```python
from build123d import *

# Parameters (mm, degrees)
ESBO_O1_R                = 14.5
RESSALTO_EXTRUS_O1_DEPTH = 17
ESBO_O1_4_R              = 14.5
ESBO_O1_4_R_2            = 4
RESSALTO_EXTRUS_O2_DEPTH = 13
RESSALTO_EXTRUS_O3_DEPTH = 5
ESBO_O1_9_R              = 4
RESSALTO_EXTRUS_O4_DEPTH = 2


with BuildPart() as part:
    # Esboço1 → Ressalto-extrusão1 (new, symmetric)
    with BuildSketch(Plane.XY):
        with BuildLine():
            ThreePointArc((-16.377431433, -13), (-16.816771262, -14.060660172), (-17.877431433, -14.5))
            Line((-17.877431433, -14.5), (-93.857447864, -14.5))
            Line((-93.857447864, -14.5), (-94.796189578, -14.5))
            ThreePointArc((-94.796189578, -14.5), (-142.377431433, 0), (-94.796189578, 14.5))
            Line((-94.796189578, 14.5), (-93.857447864, 14.5))
            Line((-93.857447864, 14.5), (-17.877431433, 14.5))
            ThreePointArc((-17.877431433, 14.5), (-16.816771262, 14.060660172), (-16.377431433, 13))
            Line((-16.377431433, 13), (-16.377431433, -13))
        make_face()
        with Locations((-116.377431433, 0)):
            Circle(ESBO_O1_R, mode=Mode.SUBTRACT)
        with BuildLine():
            ThreePointArc((-67.404246513, -2), (-55.027431433, 0), (-67.404246513, 2))
            Line((-67.404246513, 2), (-72.243354514, 2))
            Line((-72.243354514, 2), (-72.243354514, -2))
            Line((-72.243354514, -2), (-67.404246513, -2))
        make_face(mode=Mode.SUBTRACT)
    extrude(amount=RESSALTO_EXTRUS_O1_DEPTH, both=True)

    # Esboço1<4> → Ressalto-extrusão2 (add, symmetric)
    # profile 1 of 3: a face of its own
    with BuildSketch(Plane.XY):
        with BuildLine():
            Line((-17.877431433, 14.5), (-93.857447864, 14.5))
            Line((-93.857447864, 14.5), (-94.796189578, 14.5))
            ThreePointArc((-94.796189578, 14.5), (-142.377431433, 0), (-94.796189578, -14.5))
            Line((-94.796189578, -14.5), (-93.857447864, -14.5))
            Line((-93.857447864, -14.5), (-17.877431433, -14.5))
            ThreePointArc((-17.877431433, -14.5), (-16.816771262, -14.060660172), (-16.377431433, -13))
            Line((-16.377431433, -13), (-16.377431433, 13))
            ThreePointArc((-16.377431433, 13), (-16.816771262, 14.060660172), (-17.877431433, 14.5))
        make_face()
        with Locations((-116.377431433, 0)):
            Circle(ESBO_O1_4_R, mode=Mode.SUBTRACT)
        with BuildLine():
            ThreePointArc((-67.404246513, 2), (-55.027431433, 0), (-67.404246513, -2))
            Line((-67.404246513, -2), (-72.243354514, -2))
            Line((-72.243354514, -2), (-72.243354514, 2))
            Line((-72.243354514, 2), (-67.404246513, 2))
        make_face(mode=Mode.SUBTRACT)
    # profile 2 of 3: a face of its own
    with BuildSketch(Plane.XY):
        Polygon((-1.377431433, 13.000001379), (-16.377431433, 13), (-16.377431433, -13), (-1.377431433, -13), align=None)
    # profile 3 of 3: a face of its own
    with BuildSketch(Plane.XY):
        with Locations((123.619903756, 0)):
            Circle(ESBO_O1_4_R_2)
    extrude(amount=RESSALTO_EXTRUS_O2_DEPTH, both=True)


with BuildPart() as ressalto_extrus_o2_kept_piece:
    # of the separate pieces the step leaves, the one the design keeps (ressalto_extrus_o2_pieces_kept)
    add(part.part.solids().sort_by_distance((-16.377431433, -13, -17))[0])

    # Esboço1<8> → Ressalto-extrusão3 (add, symmetric)
    with BuildSketch(Plane.XY):
        with BuildLine():
            Line((123.625891638, -13), (-1.377431433, -13))
            Line((-1.377431433, -13), (-1.377431433, 13.000001379))
            Line((-1.377431433, 13.000001379), (123.619903756, 13.000001379))
            ThreePointArc((123.619903756, 13.000001379), (136.61990479, 0.002993941), (123.625891638, -13))
        make_face()
        with BuildLine():
            ThreePointArc((18.619903756, 9), (9.619903756, 0), (18.619903756, -9))
            Line((18.619903756, -9), (123.619903756, -9))
            ThreePointArc((123.619903756, -9), (132.619903756, 0), (123.619903756, 9))
            Line((123.619903756, 9), (18.619903756, 9))
        make_face(mode=Mode.SUBTRACT)
    extrude(amount=RESSALTO_EXTRUS_O3_DEPTH, both=True)

    # Esboço1<9> → Ressalto-extrusão4 (add, symmetric)
    with BuildSketch(Plane.XY):
        with BuildLine():
            Line((123.619903756, 9), (18.619903756, 9))
            ThreePointArc((18.619903756, 9), (9.619903756, 0), (18.619903756, -9))
            Line((18.619903756, -9), (123.619903756, -9))
            ThreePointArc((123.619903756, -9), (132.619903756, 0), (123.619903756, 9))
        make_face()
        with Locations((123.619903756, 0)):
            Circle(ESBO_O1_9_R, mode=Mode.SUBTRACT)
    extrude(amount=RESSALTO_EXTRUS_O4_DEPTH, both=True)


solid = ressalto_extrus_o2_kept_piece.part
```
Can you work these out from the model? Positions are in its coordinate system, mm. A direction names the side the tool comes from. Coordinates: 2 decimals unless noted, no trailing zeros. Order: outer loops, then holes, each group sorted by start corner. A loop starts at its lowest first (then second) coordinate and runs counter-clockwise, first axis right, second up.
1. If we section it at D-D (y = -20): Please give me the cut outline in (x, z), then the cut area to 3 significant figures.
2. For faces 1 (the face through (-9, 0, -13)), 2 (the face through (70, 0, -2)), 3 (the face through (37, -13, 0)), 4 (the face through (-1.377, 0, 9)), which set-ups out of +Z, -Z, +X, -X, +Y, -Y let a thin tool reach every point of the face, with its end or its side?
3. I need wall thicknesses on line 1 (Y direction, x = 46.5, z = -3); line 2 (Y direction, x = -68, z = 6.5); line 3 (Z direction, x = 26, y = -4.5). Which ranges of each line are inside material? Lowest first, please.
4. If we section it at A-A (z = -10): Please give me the cut outline in (x, y), then the cut area to 3 significant figures.
5. If we section it at C-C (x = 92): Please give me the cut outline in (y, z).
6. Thinking about a two-plate mould opening in Y: for faces 5 (the face through (9.622, 0.198, -3.479)), 6 (the face through (-1.377, 0, -9)), 7 (the face through (-57, -14.5, 0)), which applies, +Y half, -Y half, draft (parallel to the pull), parting line (faces both ways), or undercut?
7. If we section it at B-B (x = -107): Please give me the cut outline in (y, z), then the cut area to 3 significant figures.
8. I'm going to push flat-ended pins straight in: pin 1 (4.5 mm diameter, centred on x = -70.5, z = 14, fed in from +Y); pin 2 (8 mm diameter, centred on x = 54, z = -8, fed in from -Y); pin 3 (7.5 mm diameter, centred on x = -61.38, y = 0, fed in from +Z); pin 4 (4.5 mm diameter, centred on y = -3.5, z = -15.5, fed in from +X). Where does each tip first touch, or does it pass through?
Entries:
1. outline: (-132.99, -17) - (-99.76, -17) - (-99.76, 17) - (-132.99, 17) - close
1. area: 1,130 mm2
2. face 1: -Z, +X, +Y, -Y
2. face 2: -Z
2. face 3: +Z, -Z, +X, -Y
2. face 4: +Z, +X, +Y, -Y
3. line 1: y = -13 to -9, 9 to 13
3. line 2: y = -14.5 to -2, 2 to 14.5
3. line 3: z = -2 to 2
4. outline: (-94.8, -14.5) - (-17.88, -14.5) arc R1.5 ccw to (-16.38, -13) - (-1.38, -13) - (-1.38, 13) - (-16.38, 13) arc R1.5 ccw to (-17.88, 14.5) - (-94.8, 14.5) arc R26 ccw (long way) to start; hole circle Ø29 at (-116.38, 0); hole (-72.24, -2) - (-67.4, -2) arc R6.35 ccw (long way) to (-67.4, 2) - (-72.24, 2) - close
4. area: 3,890 mm2
5. outline: (-13, -5) - (-9, -5) - (-9, -2) - (9, -2) - (9, -5) - (13, -5) - (13, 5) - (9, 5) - (9, 2) - (-9, 2) - (-9, 5) - (-13, 5) - close
6. face 5: undercut
6. face 6: draft
6. face 7: -Y half
7. outline: (-24.25, -17) - (-11.06, -17) - (-11.06, 17) - (-24.25, 17) - close; (11.06, -17) - (24.25, -17) - (24.25, 17) - (11.06, 17) - close
7. area: 897 mm2
8. pin 1: stops at y = 14.5
8. pin 2: stops at y = -13
8. pin 3: passes through
8. pin 4: stops at x = -16.38
